```python
from build123d import *

# Parameters (mm, degrees)
SKETCH1_W           = 127
SKETCH1_H           = 25.4
SKETCH1_R           = 3.175
SKETCH1_R_2         = 1.5875
BOSS_EXTRUDE1_DEPTH = 3.175


with BuildPart() as part:
    # Sketch1 → Boss-Extrude1 (new body)
    with BuildSketch(Plane(origin=(0, 0, 0), x_dir=(1, 0, 0), z_dir=(0, 1, 0))):
        Rectangle(SKETCH1_W, SKETCH1_H)
        with Locations((-50.8, 0)):
            Circle(SKETCH1_R, mode=Mode.SUBTRACT)
        with Locations((50.8, 0)):
            Circle(SKETCH1_R, mode=Mode.SUBTRACT)
        with Locations((-13.774801, 0)):
            Circle(SKETCH1_R_2, mode=Mode.SUBTRACT)
        with Locations((13.774801, 0)):
            Circle(SKETCH1_R_2, mode=Mode.SUBTRACT)
    extrude(amount=BOSS_EXTRUDE1_DEPTH)


solid = part.part
```
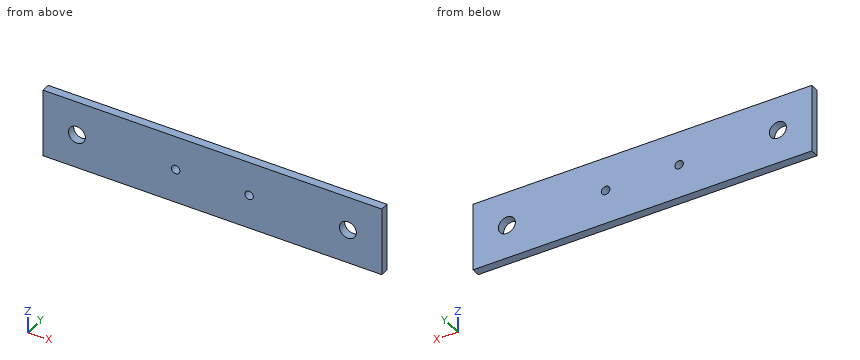
The model under review builds one solid part; all positions refer to its coordinate system, in mm. Give positions to 0.01 mm unless a question says otherwise; leave off trailing zeros. Write each loop counter-clockwise with the first axis right and the second up, starting at its lowest first coordinate (ties: lowest second). Pieces come first, ordered by that corner, then holes.
(1) Consider section C-C, the plane z = 0. Give the boundary of the cut face in (x, y) (3 decimals), and give its area (3 significant figures).
(2) Consider section A-A, the plane x = -50.8. Give the boundary of the cut face in (y, z) (3 decimals).
(3) Consider section B-B, the plane y = 0.5. Give the number of separate pieces and of enclosed holes in the cut face, and give its area (3 significant figures).
(4) To check wall thickness, follow L1, parallel to X at y = 1.95, z = 0 (3 decimals); L2, parallel to Z at x = 50.8, y = 2.5 (3 decimals); L3, parallel to X at y = 0.35, z = -0.5. State the ranges of each line that lie inside material, in increasing order.
Returned:
1. outline: (-63.5, 0) - (-53.975, 0) - (-53.975, 3.175) - (-63.5, 3.175) - close; (-47.625, 0) - (-15.362, 0) - (-15.362, 3.175) - (-47.625, 3.175) - close; (-12.187, 0) - (12.187, 0) - (12.187, 3.175) - (-12.187, 3.175) - close; (15.362, 0) - (47.625, 0) - (47.625, 3.175) - (15.362, 3.175) - close; (53.975, 0) - (63.5, 0) - (63.5, 3.175) - (53.975, 3.175) - close
1. area: 343 mm2
2. outline: (0, -12.7) - (3.175, -12.7) - (3.175, -3.175) - (0, -3.175) - close; (0, 3.175) - (3.175, 3.175) - (3.175, 12.7) - (0, 12.7) - close
3. separate pieces: 1
3. enclosed holes: 4
3. area: 3,150 mm2
4. L1: x = -63.5 to -53.975, -47.625 to -15.362, -12.187 to 12.187, 15.362 to 47.625, 53.975 to 63.5
4. L2: z = -12.7 to -3.175, 3.175 to 12.7
4. L3: x = -63.5 to -53.94, -47.66 to -15.28, -12.27 to 12.27, 15.28 to 47.66, 53.94 to 63.5
